from build123d import *

# Parameters (mm, degrees)
F0_R     = 3
F1_DEPTH = 10
F2_W     = 20
F2_H     = 8
F3_DEPTH = 2
F4_R     = 1.5
F5_DEPTH = 5
F6_R     = 2
F7_DEPTH = 1


with BuildPart() as f1:
    # F0 (on Top) → F1 (new body)
    with BuildSketch(Plane.XY):
        with BuildLine():
            ThreePointArc((-16, 5), (-19.5355339059, -3.5355339059), (-11, 0))
            ThreePointArc((-11, 0), (-12.4644660941, 3.5355339059), (-16, 5))
        make_face()
        with Locations((-16, 0)):
            Circle(F0_R, mode=Mode.SUBTRACT)
        with BuildLine():
            ThreePointArc((-16, 5), (-12.4644660941, 3.5355339059), (-11, 0))
            Line((-11, 0), (11, 0))
            ThreePointArc((11, 0), (12.4644660941, 3.5355339059), (16, 5))
            Line((16, 5), (-16, 5))
        make_face()
        with BuildLine():
            ThreePointArc((16, 5), (12.4644660941, 3.5355339059), (11, 0))
            ThreePointArc((11, 0), (16, -5), (21, 0))
            ThreePointArc((21, 0), (19.5355339059, 3.5355339059), (16, 5))
        make_face()
        with BuildLine():
            ThreePointArc((19, 0), (16, -3), (13, 0))
            ThreePointArc((13, 0), (16, 3), (19, 0))
        make_face(mode=Mode.SUBTRACT)
    extrude(amount=F1_DEPTH)

    # F2 (on face) → F3 (cut)
    with BuildSketch(Plane.XZ):
        with Locations((0, 5)):
            Rectangle(F2_W, F2_H)
    extrude(amount=-F3_DEPTH, mode=Mode.SUBTRACT)

    # F4 (on face) → F5 (cut)
    with BuildSketch(Plane(origin=(0, 5, 0), x_dir=(-1, 0, 0), z_dir=(0, 1, 0))):
        with BuildLine():
            ThreePointArc((3.5, 5), (2.4748737342, 7.4748737342), (0, 8.5))
            Line((0, 8.5), (0, 1.5))
            ThreePointArc((0, 1.5), (2.4748737342, 2.5251262658), (3.5, 5))
        make_face()
        with BuildLine():
            Line((0, 1.5), (0, 8.5))
            ThreePointArc((0, 8.5), (-3.5, 5), (0, 1.5))
        make_face()
        with Locations((6, 5)):
            Circle(F4_R)
        with Locations((-6, 5)):
            Circle(F4_R)
    extrude(amount=-F5_DEPTH, mode=Mode.SUBTRACT)

    # F6 (on face) → F7 (cut)
    with BuildSketch(Plane(origin=(0, 5, 0), x_dir=(-1, 0, 0), z_dir=(0, 1, 0))):
        with Locations((-6, 5)):
            Circle(F6_R)
        with Locations((6, 5)):
            Circle(F6_R)
    extrude(amount=-F7_DEPTH, mode=Mode.SUBTRACT)


solid = f1.part
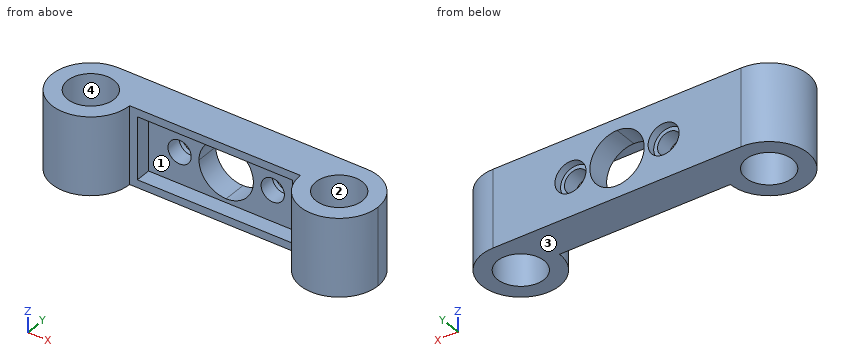
Can you work these out from the model? Positions are in its coordinate system, mm. Face numbers are marked on the shaded views. A direction names the side the tool comes from. Coordinates: 2 decimals unless noted, no trailing zeros. Write each loop counter-clockwise with the first axis right and the second up, starting at its lowest first coordinate (ties: lowest second). Pieces come first, ordered by that corner, then holes. Notation, with made-up numbers: (70.25, -4.5) -> (76.25, -4.5) arc R21 cw to (76.25, 2.5) -> close; hole circle Ø8 at (-10, 65.25). An arc over 180 degrees is marked (long way). Write each question's results on one line, items separated by ' | '. Start each with the question number.
Item 1: On a 3-axis mill with a long thin cutter (end or side, diameter ignored), from which of +Z, -Z, +X, -X, +Y, -Y can I reach the whole of each face in a straight line? I mean the marked faces 1 and 2. Say none if no direction works.
Item 2: If we section it at D-D, the plane y = 1.5: Write out the boundary of the cut face in (x, z), and give its area (3 significant figures).
Item 3: Thinking about a two-plate mould opening in X: for the marked faces 3 and 4, which applies, released by +X, released by -X, zero draft, split by the parting line, or undercut?
Item 4: If we section it at C-C, the plane x = 6: Write out the boundary of the cut face in (y, z).
Item 5: If we section it at B-B, the plane z = 4.25: Count the separate pieces of the cut face and the enclosed holes in it, and give its area (3 significant figures).
Item 6: Please list where these lines run through material, in increasing order: probe 1 along Z at (x, y) = (-6, 4.2); probe 2 along X at (y, z) = (1.75, 5.25); probe 3 along X at (y, z) = (1.5, 8).
Item 7: I'm going to push flat-ended pins straight in: P1, Ø1.6, axis at y = 1, z = 3, coming from the -X side; P2, Ø5, axis at y = 3.5, z = 5, coming from the +X side; P3, Ø2, axis at y = 3.5, z = 8.5, coming from the -X side. Where does each tip first touch, or does it pass through?
Item 8: If we section it at A-A, the plane y = -4: Write out the boundary of the cut face in (x, z), and give its area (3 significant figures).
Answer block:
1) face 1: -Y | face 2: +Z, -Z
2) outline: (-20.77, 0) -> (-18.6, 0) -> (-18.6, 10) -> (-20.77, 10) -> close; (-13.4, 0) -> (13.4, 0) -> (13.4, 10) -> (-13.4, 10) -> close; (18.6, 0) -> (20.77, 0) -> (20.77, 10) -> (18.6, 10) -> close; hole (-10, 1) -> (10, 1) -> (10, 9) -> (-10, 9) -> close | area: 151 mm²
3) face 3: zero draft | face 4: undercut
4) outline: (0, 0) -> (5, 0) -> (5, 3) -> (4, 3) -> (4, 3.5) -> (2, 3.5) -> (2, 1) -> (0, 1) -> close; (0, 9) -> (2, 9) -> (2, 6.5) -> (4, 6.5) -> (4, 7) -> (5, 7) -> (5, 10) -> (0, 10) -> close
5) separate pieces: 4 | enclosed holes: 2 | area: 143 mm²
6) probe 1: 0 to 3, 7 to 10 | probe 2: -20.68 to -18.44, -13.56 to -10, 10 to 13.56, 18.44 to 20.68 | probe 3: -20.77 to -18.6, -13.4 to -10, 10 to 13.4, 18.6 to 20.77
7) P1: x = -21 | P2: x = 20.9 | P3: x = -20.33
8) outline: (-19, 0) -> (-13, 0) -> (-13, 10) -> (-19, 10) -> close; (13, 0) -> (19, 0) -> (19, 10) -> (13, 10) -> close | area: 120 mm²
